Input: part model. Units: mm. Frame: model coordinates. A direction names the side the tool comes from. Coordinates: 2 decimals unless noted, no trailing zeros. Loops run counter-clockwise (first coordinate to the right, second up) from the corner with the lowest first, then second, coordinate; pieces in that order, holes last. Notation, with made-up numbers: (17.5, 7) -> (50.5, 7) arc R19 ccw to (50.5, 41) -> close; hole circle Ø7 at (6, 40). An arc over 180 degrees is marked (long way). Put each result on its own line as item: value. Start each with the question number.
1) Set-up query: faces 4 (the cylindrical face through (17.89, 5.49, 1.34)), 5 (the flat face through (10, 10, 0)), 6 (the flat face through (3.176, 2.465, 1.799)). Return all of +Z, -Z, +X, -X, +Y, -Y with unobstructed straight access to the full face (end or side cutting, diameter ignored); none if empty.
2) Material intervals for L1, parallel to X at y = 5.7, z = 0; L2, parallel to Z at x = 20, y = 4.05 (3 decimals); L3, parallel to Z at x = 20, y = 5.35, sorted ascending.
3) Cut plane A-A (y = 5.5). Return the cut outline in (x, z).
4) Cut plane B-B (z = -1). Return the cut outline in (x, y), plus the area to 3 significant figures.
5) Cut plane D-D (y = 7.5). Return the cut outline in (x, z).
6) Pull-direction query (X, two-part tool) for faces 1 (the cylindrical face through (-5.95, 3.82, -0.78)), 2 (the flat face through (10, 6, 6)), 3 (the flat face through (17.5, 8.03, -1.47)); classes: pulls with the +X half, pulls with the -X half, needs draft (parallel to the pull), parting line crosses it, or undercut.
7) Contact query for flat-ended pins moving along their axis: P1, Ø1, axis at y = 4.5, z = -3, coming from the +X side; P2, Ø5.5, axis at x = 20, z = 0, coming from the +Y side; P3, Ø5, axis at y = 9, z = 2, coming from the -X side; P4, Ø4, axis at x = 20, z = 0, coming from the +Y side. Output: stop coordinate, or through.
from build123d import *

# Parameters (mm, degrees)
EXTRUDE_1_DEPTH     = 10
CUT_EXTRUDE_1_DEPTH = 5
SKETCH_6_R          = 27.317981471
SKETCH_6_R_2        = 6
CUT_EXTRUDE_2_DEPTH = 2
CUT_EXTRUDE_3_DEPTH = 4


with BuildPart() as part:
    # 草图1 → 凸台-拉伸1 (new body)
    with BuildSketch(Plane(origin=(0, 0, 0), x_dir=(1, 0, 0), z_dir=(0, 1, 0))):
        with BuildLine():
            Line((0, 6), (20, 6))
            ThreePointArc((20, 6), (26, 0), (20, -6))
            Line((20, -6), (0, -6))
            ThreePointArc((0, -6), (-6, 0), (0, 6))
        make_face()
    extrude(amount=EXTRUDE_1_DEPTH)

    # 草图3 → 切除-旋转2 (revolve, cut)
    with BuildSketch(Plane.XY, mode=Mode.PRIVATE) as cut_revolve_2_sk:
        Polygon((0, 10), (-2.55, 10), (-2.55, 5), (-2.1, 5), (-2.1, 2), (-2.55, 2), (-2.55, 0), (0, 0), align=None)
    revolve(cut_revolve_2_sk.sketch.rotate(Axis((0, 10, 0), (0, -1, 0)), 270), axis=Axis((0, 10, 0), (0, -1, 0)), mode=Mode.SUBTRACT)

    # 草图4 → 切除-旋转3 (revolve, cut)
    with BuildSketch(Plane.XY, mode=Mode.PRIVATE) as cut_revolve_3_sk:
        Polygon((20, 10), (17.5, 10), (17.5, 5), (17.925, 5), (17.925, 0), (20, 0), align=None)
    revolve(cut_revolve_3_sk.sketch.rotate(Axis((20, 10, 0), (0, -1, 0)), 270), axis=Axis((20, 10, 0), (0, -1, 0)), mode=Mode.SUBTRACT)

    # 草图5 → 切除-拉伸1 (cut)
    with BuildSketch(Plane.XZ):
        Polygon((-4.214656965, 0), (-2.107328483, -3.65), (2.107328483, -3.65), (4.214656965, 0), (2.107328483, 3.65), (-2.107328483, 3.65), align=None)
    extrude(amount=-CUT_EXTRUDE_1_DEPTH, mode=Mode.SUBTRACT)

    # 草图6 → 切除-拉伸2 (cut)
    with BuildSketch(Plane.XZ):
        Circle(SKETCH_6_R)
        with Locations(Location((0, 0, 0), (0, 0, 90))):
            Circle(SKETCH_6_R_2, mode=Mode.SUBTRACT)
    extrude(amount=-CUT_EXTRUDE_2_DEPTH, mode=Mode.SUBTRACT)

    # 草图7 → 切除-拉伸3 (cut)
    with BuildSketch(Plane(origin=(0, 10, 0), x_dir=(1, 0, 0), z_dir=(0, 1, 0))):
        Polygon((18.325684219, 2.9), (16.651368439, 0), (18.325684219, -2.9), (21.674315781, -2.9), (23.348631561, 0), (21.674315781, 2.9), align=None)
    extrude(amount=-CUT_EXTRUDE_3_DEPTH, mode=Mode.SUBTRACT)


solid = part.part
Results found:
1. face 4: +Y
1. face 5: +Z, -Z, +X, -X, +Y
1. face 6: -Y
2. L1: x = -6 to -2.55, 2.55 to 17.5, 22.5 to 26
2. L2: z = -6 to -2.075, 2.075 to 6
2. L3: z = -6 to -2.5, 2.5 to 6
3. outline: (0, -6) -> (20, -6) arc R6 ccw to (20, 6) -> (0, 6) arc R6 ccw to start; hole circle Ø5.1 at (0, 0); hole circle Ø5 at (20, 0)
4. outline: (-5.92, 0) -> (-3.64, 0) -> (-3.64, 5) -> (-2.35, 5) -> (-2.35, 10) -> (-5.92, 10) -> close; (2.35, 5) -> (3.64, 5) -> (3.64, 0) -> (5.92, 0) -> (5.92, 2) -> (18.18, 2) -> (18.18, 5) -> (17.71, 5) -> (17.71, 6) -> (17.23, 6) -> (17.23, 10) -> (2.35, 10) -> close; (21.82, 2) -> (25.92, 2) -> (25.92, 10) -> (22.77, 10) -> (22.77, 6) -> (22.29, 6) -> (22.29, 5) -> (21.82, 5) -> close
4. area: 181 mm2
5. outline: (0, -6) -> (20, -6) arc R6 ccw to (20, 6) -> (0, 6) arc R6 ccw to start; hole circle Ø5.1 at (0, 0); hole (16.65, 0) -> (18.33, -2.9) -> (21.67, -2.9) -> (23.35, 0) -> (21.67, 2.9) -> (18.33, 2.9) -> close
6. face 1: parting line crosses it
6. face 2: needs draft
6. face 3: undercut
7. P1: stops at x = 25.45
7. P2: stops at y = 6
7. P3: stops at x = -6
7. P4: passes through
